Can you work these out from the model? Positions are in its coordinate system, mm. Face numbers are marked on the shaded views. A direction names the side the tool comes from. Give positions to 0.01 mm unless a question says otherwise; leave off trailing zeros. Order: outer loops, then holes, each group sorted by start corner. A loop starts at its lowest first (then second) coordinate and runs counter-clockwise, first axis right, second up.
Item 1: Which directions (+Z, -Z, +X, -X, +Y, -Y) give clear straight access to the entire face, cutting with the end or side of a thin tool? Please do the marked faces 1 and 2.
Item 2: I want a section at D-D, the plane y = 21.5. Write out the boundary of the cut face in (x, z).
Item 3: I want a section at C-C, the plane x = 17. Write out the boundary of the cut face in (y, z), then the cut area to 3 significant figures.
Item 4: I want a section at B-B, the plane x = 29. Write out the boundary of the cut face in (y, z), then the cut area to 3 significant figures.
Item 5: If I drill on line 1 along X through (y, z) = (4.3, -21.25); line 2 along Y through (x, z) = (-10.5, -37.85); line 3 along Y through (x, z) = (-10, -36), over which ranges is the centre line in solid material (lowest first)?
Item 6: I want a section at A-A, the plane z = 27.75. Write out the boundary of the cut face in (x, y), then the cut area to 3 significant figures.
Item 7: I'm going to push flat-ended pins straight in: pin 1 Ø1.5 at (x, z) = (28.5, -21.5) entering from +Y; pin 2 Ø2 at (x, z) = (-1, -32) entering from +Y; pin 3 Ø10 at (x, z) = (34, -3.5) entering from +Y. Where does each tip first touch, or does it pass through?
```python
from build123d import *

# Parameters (mm, degrees)
SKETCH1_W                 = 100
SKETCH1_H                 = 70
BOSS_EXTRUDE1_DEPTH       = 3
SKETCH2_W                 = 100
SKETCH2_H                 = 6.5
BOSS_EXTRUDE2_DEPTH       = 30
SKETCH14_R                = 2.5
BOSS_EXTRUDE5_DEPTH       = 3
F_2_5MM_DOWEL_HOLE4_D     = 2.5
SKETCH21_W                = 30
SKETCH21_H                = 4
BOSS_EXTRUDE6_DEPTH       = 4
SKETCH22_W                = 30
SKETCH22_H                = 4
BOSS_EXTRUDE7_DEPTH       = 30
FILLET6_R                 = 4
FILLET7_R                 = 4
FILLET8_R                 = 4
M2X0_4_TAPPED_HOLE1_D     = 1.6
M2X0_4_TAPPED_HOLE1_DEPTH = 13
M2X0_4_TAPPED_HOLE1_TIP   = 0.480688495
FILLET9_R                 = 4
CUT_EXTRUDE10_DEPTH       = 14


with BuildPart() as part:
    # Sketch1 → Boss-Extrude1 (new body)
    with BuildSketch(Plane(origin=(0, 0, 0), x_dir=(1, 0, 0), z_dir=(0, 1, 0))):
        Rectangle(SKETCH1_W, SKETCH1_H)
    extrude(amount=BOSS_EXTRUDE1_DEPTH)

    # Sketch2 → Boss-Extrude2 (add)
    with BuildSketch(Plane(origin=(0, 3, 0), x_dir=(1, 0, 0), z_dir=(0, 1, 0))):
        with Locations((0, 31.75)):
            Rectangle(SKETCH2_W, SKETCH2_H)
    extrude(amount=BOSS_EXTRUDE2_DEPTH)

    # Sketch14 → Boss-Extrude5 (add)
    with BuildSketch(Plane(origin=(0, 3, -3), x_dir=(1, 0, 0), z_dir=(0, -1, 0))):
        with Locations(Location((-29, -18.25, 0), (0, 0, 270))):
            Circle(SKETCH14_R)
        with Locations(Location((-29, 30.75, 0), (0, 0, 270))):
            Circle(SKETCH14_R)
        with Locations(Location((29, -18.25, 0), (0, 0, 270))):
            Circle(SKETCH14_R)
        with Locations(Location((29, 30.75, 0), (0, 0, 270))):
            Circle(SKETCH14_R)
    extrude(amount=-BOSS_EXTRUDE5_DEPTH)

    # Ø2.5mm Dowel Hole4 (through all)
    with Locations(Plane(origin=(0, 6, 0), x_dir=(1, 0, 0), z_dir=(0, 1, 0))):
        with Locations((-29, 21.25), (29, 21.25), (29, -27.75), (-29, -27.75)):
            Hole(F_2_5MM_DOWEL_HOLE4_D / 2)

    # Sketch21 → Boss-Extrude6 (add)
    with BuildSketch(Plane(origin=(0, 0, -35), x_dir=(-1, 0, 0), z_dir=(0, 0, -1))):
        with Locations((0, 31)):
            Rectangle(SKETCH21_W, SKETCH21_H)
    extrude(amount=BOSS_EXTRUDE6_DEPTH)

    # Sketch22 → Boss-Extrude7 (add)
    with BuildSketch(Plane(origin=(0, 33, 0), x_dir=(1, 0, 0), z_dir=(0, 1, 0))):
        with Locations((0, 37)):
            Rectangle(SKETCH22_W, SKETCH22_H)
    extrude(amount=BOSS_EXTRUDE7_DEPTH)

    # Fillet6
    fillet6_edges = [part.edges().sort_by_distance(p)[0] for p in [
        (0, 33, -35),
    ]]
    fillet(fillet6_edges, radius=FILLET6_R)

    # Fillet7
    fillet7_edges = [part.edges().sort_by_distance(p)[0] for p in [
        (0, 29, -35),
    ]]
    fillet(fillet7_edges, radius=FILLET7_R - 0.0001)  # a hair under: the kernel refuses the full size

    # Fillet8
    fillet8_edges = [part.edges().sort_by_distance(p)[0] for p in [
        (0, 29, -39),
    ]]
    fillet(fillet8_edges, radius=FILLET8_R)

    # M2x0.4 Tapped Hole1
    with Locations(Plane(origin=(0, 0, -39), x_dir=(-1, 0, 0), z_dir=(0, 0, -1))):
        with Locations((-10.5, 56.728604695), (10.5, 56.728604695), (10.5, 44.228604695), (-10.5, 44.228604695)):
            Hole(M2X0_4_TAPPED_HOLE1_D / 2, depth=M2X0_4_TAPPED_HOLE1_DEPTH)
            with Locations((0, 0, -(M2X0_4_TAPPED_HOLE1_DEPTH + M2X0_4_TAPPED_HOLE1_TIP / 2))):  # 118° drill point
                Cone(0, M2X0_4_TAPPED_HOLE1_D / 2, M2X0_4_TAPPED_HOLE1_TIP, mode=Mode.SUBTRACT)

    # Fillet9
    fillet9_edges = [part.edges().sort_by_distance(p)[0] for p in [
        (0, 3, -28.5),
    ]]
    fillet(fillet9_edges, radius=FILLET9_R)

    # Sketch28 → Cut-Extrude10 (cut)
    with BuildSketch(Plane.XY.offset(-28.5)):
        with BuildLine():
            Line((-20, 25.135697653), (20, 25.135697653))
            ThreePointArc((20, 25.135697653), (25.424121319, 19.711576334), (20, 14.287455015))
            Line((20, 14.287455015), (-20, 14.287455015))
            ThreePointArc((-20, 14.287455015), (-25.424121319, 19.711576334), (-20, 25.135697653))
        make_face()
    extrude(amount=-CUT_EXTRUDE10_DEPTH, mode=Mode.SUBTRACT)


solid = part.part
```
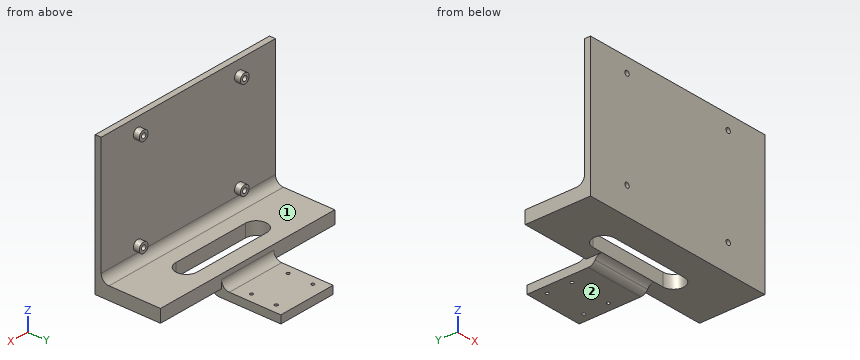
Results list:
1. face 1: +Z, +X, -X, +Y
1. face 2: -Z, +X, -X, +Y, -Y
2. outline: (-50, -35) - (-25.12, -35) - (-25.12, -28.5) - (-50, -28.5) - close; (25.12, -35) - (50, -35) - (50, -28.5) - (25.12, -28.5) - close
3. outline: (0, -35) - (14.29, -35) - (14.29, -28.5) - (7, -28.5) arc R4 cw to (3, -24.5) - (3, 35) - (0, 35) - close; (25.14, -35) - (33, -35) - (33, -28.5) - (25.14, -28.5) - close
3. area: 338 mm2
4. outline: (0, -35) - (33, -35) - (33, -28.5) - (7, -28.5) arc R4 cw to (3, -24.5) - (3, -23.75) - (6, -23.75) - (6, -22.5) - (0, -22.5) - close; (0, -20) - (6, -20) - (6, -18.75) - (3, -18.75) - (3, 25.25) - (6, 25.25) - (6, 26.5) - (0, 26.5) - close; (0, 29) - (6, 29) - (6, 30.25) - (3, 30.25) - (3, 35) - (0, 35) - close
4. area: 408 mm2
5. line 1: x = -31.5 to -30.25, -27.75 to -26.5, 26.5 to 27.75, 30.25 to 31.5
5. line 2: y = 29.12 to 43.43, 45.03 to 55.93, 57.53 to 63
5. line 3: y = 27.65 to 43.6, 44.85 to 56.1, 57.35 to 63
6. outline: (-50, 0) - (-30.25, 0) - (-30.25, 6) - (-31.5, 6) - (-31.5, 3) - (-50, 3) - close; (-27.75, 0) - (27.75, 0) - (27.75, 6) - (26.5, 6) - (26.5, 3) - (-26.5, 3) - (-26.5, 6) - (-27.75, 6) - close; (30.25, 0) - (50, 0) - (50, 3) - (31.5, 3) - (31.5, 6) - (30.25, 6) - close
6. area: 300 mm2
7. pin 1: stops at y = 6
7. pin 2: stops at y = 33.54
7. pin 3: stops at y = 3
